```python
from build123d import *

# Parameters (mm, degrees)
F0_R      = 6.35
F1_DEPTH  = 5.588
F2_SIZE   = 5.08
F1_FACE_R = 1.27
F3_DEPTH  = 66.675


with BuildPart() as f1:
    # F0 (on Top) → F1 (new body)
    with BuildSketch(Plane.XY):
        Circle(F0_R)
    extrude(amount=F1_DEPTH)

    # F2
    f2_edges = [f1.edges().sort_by_distance(p)[0] for p in [
        (-6.35, 0, 5.588),
    ]]
    chamfer(f2_edges, length=F2_SIZE)

    # F1_face (on face) → F3 (join)
    with BuildSketch(Plane.XY.offset(5.588)):
        Circle(F1_FACE_R)
    extrude(amount=F3_DEPTH)


solid = f1.part
```
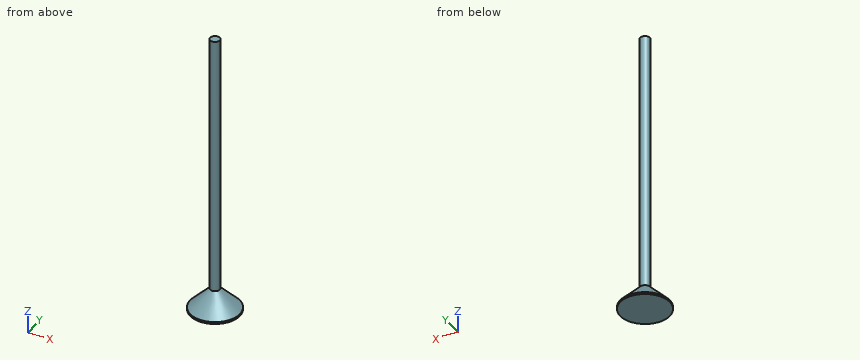
Geometry: final body of the model. Coordinates: model frame, mm. Round coordinates to 2 decimals unless told otherwise and drop trailing zeros. Order: outer loops, then holes, each group sorted by start corner. A loop starts at its lowest first (then second) coordinate and runs counter-clockwise, first axis right, second up. Notation, with made-up numbers: (51.25, -25.5) - (100.25, -25.5) arc R27 cw to (100.25, -5.5) - close; hole circle Ø4 at (51.5, 66). An arc over 180 degrees is marked (long way). Use CSV: the item, a comma, the result in double quotes. Start each with the question number.
Q1. Section query C-C (z = 52). Return loops of the section in (x, y).
Q2. Material intervals for line 1 along Z through (x, y) = (2, -5.25); line 2 along Z through (x, y) = (-3.5, 0.5); line 3 along X through (y, z) = (0.5, 48), sorted ascending. Write a range as from..to.
Q3. Section query A-A (x = 0). Return loops of the section in (y, z).
Q4. First-contact query: pin 1 (1 mm diameter, centred on y = 1.5, z = 18, fed in from -X); pin 2 (5 mm diameter, centred on y = 2.5, z = 10, fed in from +X); pin 3 (6 mm diameter, centred on y = 5, z = 64, fed in from +X); pin 4 (3 mm diameter, centred on x = -0.5, z = 31, fed in from +Y). Flat tips, straight axial feed; report the tip coordinate or a pass-through.
Result set:
1,outline,"circle Ø2.54 at (0, 0)"
2,line 1,"z = 0..1.24"
2,line 2,"z = 0..3.32"
2,line 3,"x = -1.17..1.17"
3,outline,"(-6.35, 0) - (6.35, 0) - (6.35, 0.51) - (1.27, 5.59) - (1.27, 72.26) - (-1.27, 72.26) - (-1.27, 5.59) - (-6.35, 0.51) - close"
4,pin 1,"stops at x = -0.78"
4,pin 2,"stops at x = 1.27"
4,pin 3,"passes through"
4,pin 4,"stops at y = 1.27"
